```python
from build123d import *

# Parameters (mm, degrees)
SKETCH1_R             = 10.975
SKETCH1_R_2           = 9.775
BOSS_EXTRUDE1_DEPTH   = 3.5
SKETCH1_R_3           = 5.81
SKETCH1_R_4           = 4.025
BOSS_EXTRUDE1_2_DEPTH = 3.5
SKETCH1_3_R           = 9.775
SKETCH1_3_R_2         = 5.81
BOSS_EXTRUDE2_DEPTH   = 3.25
CHAMFER1_SIZE         = 0.25
CHAMFER2_SIZE         = 0.25
CHAMFER3_SIZE         = 0.25


with BuildPart() as part:
    # Sketch1 → Boss-Extrude1 (new body, symmetric)
    with BuildSketch(Plane(origin=(0, 0, 0), x_dir=(1, 0, 0), z_dir=(0, 1, 0))):
        Circle(SKETCH1_R)
        Circle(SKETCH1_R_2, mode=Mode.SUBTRACT)
    extrude(amount=BOSS_EXTRUDE1_DEPTH, both=True)

    # Chamfer2
    chamfer2_edges = [part.edges().sort_by_distance(p)[0] for p in [
        (-10.975, 3.5, 0),
        (-10.975, -3.5, 0),
        (-9.775, -3.5, 0),
        (-9.775, 3.5, 0),
    ]]
    chamfer(chamfer2_edges, length=CHAMFER2_SIZE)


with BuildPart() as body_2:
    # Sketch1 → Boss-Extrude1 2 (new body, symmetric)
    with BuildSketch(Plane(origin=(0, 0, 0), x_dir=(1, 0, 0), z_dir=(0, 1, 0))):
        Circle(SKETCH1_R_3)
        Circle(SKETCH1_R_4, mode=Mode.SUBTRACT)
    extrude(amount=BOSS_EXTRUDE1_2_DEPTH, both=True)

    # Chamfer3
    chamfer3_edges = [body_2.edges().sort_by_distance(p)[0] for p in [
        (-5.81, 3.5, 0),
        (-5.81, -3.5, 0),
        (-4.025, -3.5, 0),
        (-4.025, 3.5, 0),
    ]]
    chamfer(chamfer3_edges, length=CHAMFER3_SIZE)


with BuildPart() as body_3:
    # Sketch1<3> → Boss-Extrude2 (new body, symmetric)
    with BuildSketch(Plane(origin=(0, 0, 0), x_dir=(1, 0, 0), z_dir=(0, 1, 0))):
        Circle(SKETCH1_3_R)
        Circle(SKETCH1_3_R_2, mode=Mode.SUBTRACT)
    extrude(amount=BOSS_EXTRUDE2_DEPTH, both=True)

    # Chamfer1
    chamfer1_edges = [body_3.edges().sort_by_distance(p)[0] for p in [
        (-9.775, 3.25, 0),
        (-9.775, -3.25, 0),
        (-5.81, -3.25, 0),
        (-5.81, 3.25, 0),
    ]]
    chamfer(chamfer1_edges, length=CHAMFER1_SIZE)

    # Combine1: union body 2, part
    add(body_2.part)
    add(part.part)


solid = body_3.part
```
Check sheet for the modelled part. Datum: model origin and axes. Units: mm. Round coordinates to 2 decimals unless told otherwise and drop trailing zeros. Order: outer loops, then holes, each group sorted by start corner. A loop starts at its lowest first (then second) coordinate and runs counter-clockwise, first axis right, second up. Notation, with made-up numbers: M 36,80 L 88,80 A26 cw 88,119 Z; hole C 4.25,45.5 d5. An arc over 180 degrees is marked long. Answer in a Markdown table with one row per item.
(1) Material ranges on line 1 along X through (y, z) = (1.5, 0) (3 decimals); line 2 along Z through (x, y) = (0, 3.2) (3 decimals), recorded low to high. Write a range as from..to.
Findings:
| item | result |
|---|---|
| line 1 | x = -10.975..-4.025, 4.025..10.975 |
| line 2 | z = -10.975..-9.775, -9.575..-6.01, -5.81..-4.025, 4.025..5.81, 6.01..9.575, 9.775..10.975 |
(2) Draft check along Z on faces 1 (the cylindrical face through (-1.43, 0.05, -10.88)), 2 (the flat face through (-0.13, -3.25, 6.22)), 3 (the flat face through (-0.13, 3.25, 6.22)), 4 (the flat face through (2, 3.5, 4)). Enter one of: +Z half, -Z half, draft (parallel to the pull), parting line (faces both ways), or undercut.
Findings:
| item | result |
|---|---|
| face 1 | parting line |
| face 2 | undercut |
| face 3 | undercut |
| face 4 | draft |
(3) Gauge pin test, flat ends, axial feed: pin 1 (4 mm diameter, centred on x = -5, y = 0, fed in from +Z); pin 2 (8 mm diameter, centred on x = -8, z = 5.5, fed in from +Y); pin 3 (1 mm diameter, centred on x = -2, y = 2.5, fed in from -Z); pin 4 (1.5 mm diameter, centred on x = -3, y = -2, fed in from +Z). Record the tip position at first contact, or that the pin passes through.
Findings:
| item | result |
|---|---|
| pin 1 | stops at z = 10.56 |
| pin 2 | stops at y = 3.5 |
| pin 3 | stops at z = -10.87 |
| pin 4 | stops at z = 10.74 |
(4) Section check A-A on y = 0. Record the boundary of the cut face in (x, z) (3 decimals), plus the area to 3 significant figures.
Findings:
| item | result |
|---|---|
| outline | C 0,0 d21.95; hole C 0,0 d8.05 |
| area | 328 mm^2 |
